Work out the finished part from the listing and answer in its coordinate system (mm). Give positions to 0.01 mm unless a question says otherwise; leave off trailing zeros. Loops run counter-clockwise (first coordinate to the right, second up) from the corner with the lowest first, then second, coordinate; pieces in that order, holes last. Notation, with made-up numbers: (75.5, 32) - (125.5, 32) arc R18 cw to (125.5, 66) - close; hole circle Ø5 at (15, 73). An arc over 180 degrees is marked (long way). One line per item, written item: value.
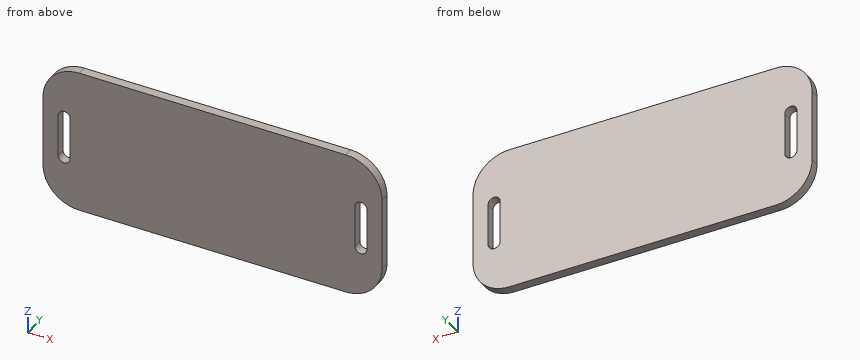
from build123d import *

# Parameters (mm, degrees)
BOSS_EXTRUDE1_DEPTH = 19.05
CUT_EXTRUDE2_DEPTH  = 388.35


with BuildPart() as part:
    # Sketch1 → Boss-Extrude1 (new body)
    with BuildSketch(Plane(origin=(0, 0, 0), x_dir=(1, 0, 0), z_dir=(0, 1, 0))):
        with BuildLine():
            Line((-279.4, 152.4), (279.4, 152.4))
            ThreePointArc((279.4, 152.4), (333.281536726, 130.081536726), (355.6, 76.2))
            Line((355.6, 76.2), (355.6, -76.2))
            ThreePointArc((355.6, -76.2), (333.281536726, -130.081536726), (279.4, -152.4))
            Line((279.4, -152.4), (-279.4, -152.4))
            ThreePointArc((-279.4, -152.4), (-333.281536726, -130.081536726), (-355.6, -76.2))
            Line((-355.6, -76.2), (-355.6, 76.2))
            ThreePointArc((-355.6, 76.2), (-333.281536726, 130.081536726), (-279.4, 152.4))
        make_face()
    extrude(amount=BOSS_EXTRUDE1_DEPTH)

    # Sketch3 → Cut-Extrude2 (cut, through all)
    with BuildSketch(Plane(origin=(0, 19.05, 0), x_dir=(1, 0, 0), z_dir=(0, 1, 0))):
        with BuildLine():
            Line((323.85, 44.45), (323.85, -44.45))
            ThreePointArc((323.85, -44.45), (311.15, -57.15), (298.45, -44.45))
            Line((298.45, -44.45), (298.45, 44.45))
            ThreePointArc((298.45, 44.45), (311.15, 57.15), (323.85, 44.45))
        make_face()
    cut_extrude2 = extrude(amount=-CUT_EXTRUDE2_DEPTH, mode=Mode.SUBTRACT)

    # Mirror1: Cut-Extrude2 across plane
    add(cut_extrude2.mirror(Plane(origin=(0, 0, 0), x_dir=(0, 0, 1), z_dir=(1, 0, 0))), mode=Mode.SUBTRACT)


solid = part.part
1. A flat-ended cylindrical pin translates along its axis: pin 1 Ø10 at (y, z) = (9, 109.5) entering from +X. Find the tip coordinate at first contact, or state that the pin passes through.
Output:
pin 1: stops at x = 350.15
2. Section C-C (x = 311.15) is taken. Write down the section's boundary in (y, z), and give its area (4 significant figures).
Output:
outline: (0, -145.47) - (19.05, -145.47) - (19.05, -57.15) - (0, -57.15) - close; (0, 57.15) - (19.05, 57.15) - (19.05, 145.47) - (0, 145.47) - close
area: 3,365 mm²
3. Section A-A (z = -1) is taken. Write down the section's boundary in (x, y), and give its area (3 significant figures).
Output:
outline: (-355.6, 0) - (-323.85, 0) - (-323.85, 19.05) - (-355.6, 19.05) - close; (-298.45, 0) - (298.45, 0) - (298.45, 19.05) - (-298.45, 19.05) - close; (323.85, 0) - (355.6, 0) - (355.6, 19.05) - (323.85, 19.05) - close
area: 12,600 mm²
4. Section D-D (z = -113.5) is taken. Write down the section's boundary in (x, y), and give its area (3 significant figures).
Output:
outline: (-345.85, 0) - (345.85, 0) - (345.85, 19.05) - (-345.85, 19.05) - close
area: 13,200 mm²
5. Find the intervals of material crossed by line 1 along X through (y, z) = (1, 17.5); line 2 along X through (y, z) = (16, 89.5); line 3 along X through (y, z) = (3.75, 110), in increasing order.
Output:
line 1: x = -355.6 to -323.85, -298.45 to 298.45, 323.85 to 355.6
line 2: x = -354.43 to 354.43
line 3: x = -347.69 to 347.69
6. Section B-B (y = 9.5) is taken. Write down the section's boundary in (x, z).
Output:
outline: (-355.6, -76.2) arc R76.2 ccw to (-279.4, -152.4) - (279.4, -152.4) arc R76.2 ccw to (355.6, -76.2) - (355.6, 76.2) arc R76.2 ccw to (279.4, 152.4) - (-279.4, 152.4) arc R76.2 ccw to (-355.6, 76.2) - close; hole (-323.85, -44.45) arc R12.7 ccw to (-298.45, -44.45) - (-298.45, 44.45) arc R12.7 ccw to (-323.85, 44.45) - close; hole (298.45, -44.45) arc R12.7 ccw to (323.85, -44.45) - (323.85, 44.45) arc R12.7 ccw to (298.45, 44.45) - close
